Input: part model. Units: mm. Frame: model coordinates. A direction names the side the tool comes from. Round coordinates to 2 decimals unless told otherwise and drop trailing zeros. Loops run counter-clockwise (first coordinate to the right, second up) from the corner with the lowest first, then second, coordinate; pieces in that order, holes last.
(1) Cut plane B-B, the plane y = 0. Output: boundary loops of the cut face in (x, z).
(2) Cut plane C-C, the plane y = 12. Output: boundary loops of the cut face in (x, z).
(3) Draft query along Z for faces 1 (the face through (6, 0, 20)), 2 (the face through (6.08, -6.85, -18.79)), 3 (the face through (5.916, -7.762, -13.415)). Return one class per face: released by +Z, released by -Z, zero draft, split by the parting line, or undercut.
(4) Cut plane D-D, the plane z = 14.5. Output: boundary loops of the cut face in (x, y), and give its area (3 significant figures).
(5) Access query for faces 4 (the face through (5.92, -12.57, -12.65)), 5 (the face through (5.92, 10.27, -14.57)), 6 (the face through (5.92, 12.57, 12.65)), 7 (the face through (6.084, -19.695, 3.48)), 8 (the face through (5.92, -17.24, 4.56)). Directions: +Z, -Z, +X, -X, +Y, -Y. A direction counts if a zero-diameter tool reaches every point of the face in a straight line with its end or side. Return the directions, or none.
(6) Line query: line 1 (Z direction, x = 8.5, y = 0); line 2 (Z direction, x = 10.75, y = -16); line 3 (Y direction, x = 8, z = 14). Output: solid intervals per line, ascending.
(7) Cut plane A-A, the plane z = 0. Output: boundary loops of the cut face in (x, y), and give its area (3 significant figures).
(8) First-contact query: pin 1 Ø4 at (x, z) = (9, -13) entering from +Y; pin 2 Ø1.5 at (x, z) = (9, -1) entering from -Y; pin 3 Ø1 at (x, z) = (2, 5.5) entering from +Y. Flat tips, straight axial feed; report the tip coordinate or a pass-through.
from build123d import *

# Parameters (mm, degrees)
BASPROSKE_W              = 12
BASPROSKE_H              = 20
TOOTHCUT_DEPTH           = 31.724582991
TEETHCUTS_COUNT          = 18
TEETHCUTS_ANGLE          = 340
BORSKE_R                 = 0.1
BORE_DEPTH               = 50.0000508
TAGLIO_ESTRUSIONE1_DEPTH = 13


with BuildPart() as part:
    # BasProSke → Base-Revolve (revolve)
    with BuildSketch(Plane(origin=(0, 0, 0), x_dir=(1, 0, 0), z_dir=(0, 1, 0)), mode=Mode.PRIVATE) as base_revolve_sk:
        with Locations((6, 10)):
            Rectangle(BASPROSKE_W, BASPROSKE_H)
    revolve(base_revolve_sk.sketch.rotate(Axis((-10, 0, 0), (1, 0, 0)), 180), axis=Axis((-10, 0, 0), (1, 0, 0)))

    # TooCutSke → ToothCut (cut, through all)
    with BuildSketch(Plane(origin=(0, 0, 0), x_dir=(0, 0, -1), z_dir=(1, 0, 0))):
        with BuildLine():
            ThreePointArc((1.007799284, 15.466199973), (0, 15.499), (-1.007799284, 15.466199973))
            ThreePointArc((-1.007799284, 15.466199973), (-1.630454606, 17.802374148), (-2.991345877, 19.800719558))
            ThreePointArc((-2.991345877, 19.800719558), (0, 20.0254), (2.991345877, 19.800719558))
            ThreePointArc((2.991345877, 19.800719558), (1.630454606, 17.802374148), (1.007799284, 15.466199973))
        make_face()
    toothcut = extrude(amount=TOOTHCUT_DEPTH, mode=Mode.SUBTRACT)

    # TeethCuts: ToothCut ×18 about axis
    teethcuts_axis = Axis((-10, 0, 0), (1, 0, 0))
    for i in range(1, TEETHCUTS_COUNT):
        add(toothcut.rotate(teethcuts_axis, i * TEETHCUTS_ANGLE / (TEETHCUTS_COUNT - 1)), mode=Mode.SUBTRACT)

    # BorSke → Bore (cut, symmetric)
    with BuildSketch(Plane(origin=(0, 0, 0), x_dir=(0, 0, -1), z_dir=(1, 0, 0))):
        with Locations(Location((0, 0, 0), (0, 0, 180))):
            Circle(BORSKE_R)
    extrude(amount=BORE_DEPTH, both=True, mode=Mode.SUBTRACT)

    # Schizzo1 → Taglio-Estrusione1 (cut)
    with BuildSketch(Plane.ZY):
        with BuildLine():
            Line((-2, 1.5), (-2, -1.5))
            ThreePointArc((-2, -1.5), (2.5, 0), (-2, 1.5))
        make_face()
    extrude(amount=-TAGLIO_ESTRUSIONE1_DEPTH, mode=Mode.SUBTRACT)


solid = part.part
Reported:
1. outline: (0, -20) - (12, -20) - (12, -2) - (0, -2) - close; (0, 2.5) - (12, 2.5) - (12, 20) - (0, 20) - close
2. outline: (0, -15.49) - (12, -15.49) - (12, -11.68) - (0, -11.68) - close; (0, -9.81) - (12, -9.81) - (12, 9.81) - (0, 9.81) - close; (0, 11.68) - (12, 11.68) - (12, 15.49) - (0, 15.49) - close
3. face 1: released by +Z
3. face 2: released by -Z
3. face 3: undercut
4. outline: (0, -13.17) - (12, -13.17) - (12, -10.17) - (0, -10.17) - close; (0, -7.11) - (12, -7.11) - (12, 7.11) - (0, 7.11) - close; (0, 10.17) - (12, 10.17) - (12, 13.17) - (0, 13.17) - close
4. area: 242 mm2
5. face 4: +X, -X, -Y
5. face 5: -Z, +X, -X
5. face 6: +X, -X, +Y
5. face 7: +Z, +X, -X, -Y
5. face 8: +X, -X
6. line 1: z = -20 to -2, 2.5 to 20
6. line 2: z = -10.43 to -7.46, -4.54 to -1.08, 1.08 to 4.54, 7.46 to 10.43
6. line 3: y = -13.06 to -9.58, -6.91 to 6.91, 9.58 to 13.06
7. outline: (0, -15.5) - (12, -15.5) - (12, -2.5) - (0, -2.5) - close; (0, 2.5) - (12, 2.5) - (12, 15.5) - (0, 15.5) - close
7. area: 312 mm2
8. pin 1: stops at y = 13.24
8. pin 2: stops at y = -18.05
8. pin 3: stops at y = 14.67
